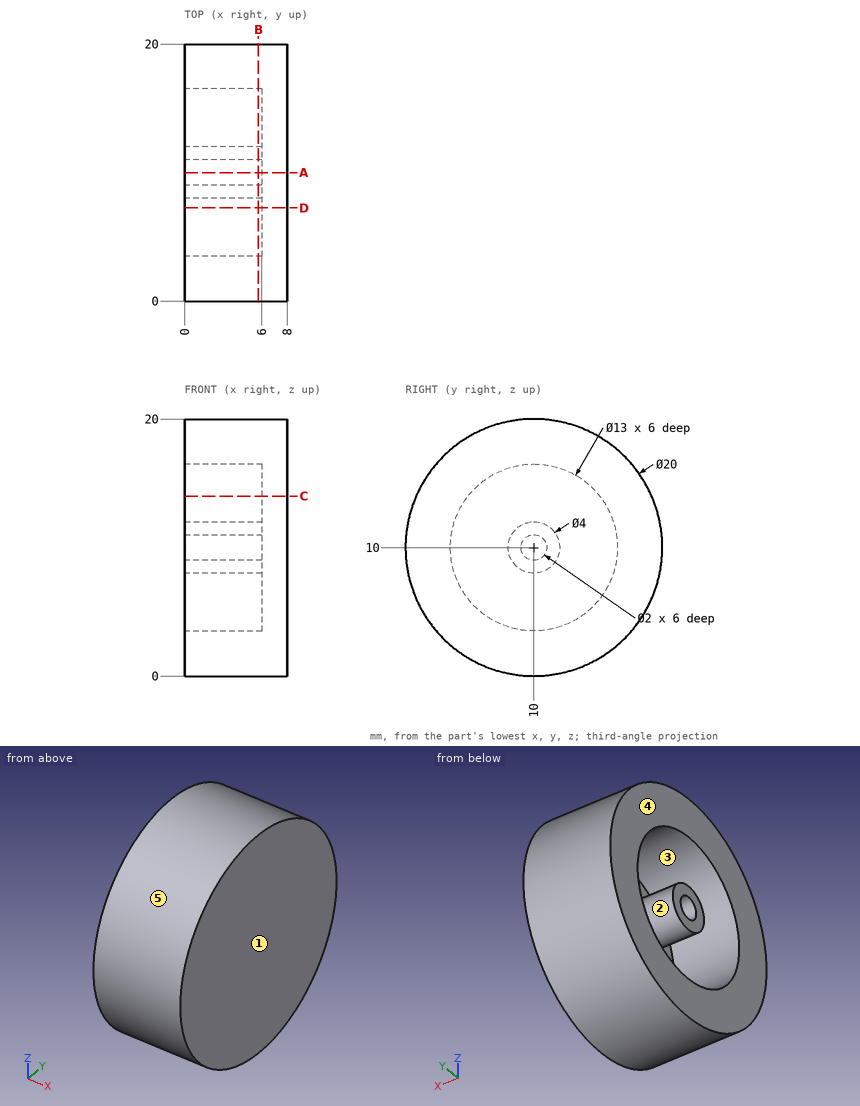
The figure shows three views and two pictorial views of one solid part (mm, origin at its lowest corner). Answer the questions. A direction names the side the tool comes from. Coordinates: 2 decimals unless noted, no trailing zeros. Order: outer loops, then holes, each group sorted by start corner. A loop starts at its lowest first (then second) coordinate and runs counter-clockwise, first axis right, second up. Notation, with made-up numbers: M 47,26 L 104,26 A7 cw 104,30 Z; hole C 69,-18.5 d4. An arc over 180 degrees is marked long. Use CSV: the item, a comma, the result in double quotes.
1) Section C-C on z = 14 is taken. Write down the section's boundary in (x, y), plus the area to 3 significant figures.
Worked out:
outline,"M 0,0.83 L 8,0.83 L 8,19.17 L 0,19.17 L 0,15.12 L 6,15.12 L 6,4.88 L 0,4.88 Z"
area,"85.2 mm^2"
2) Section B-B on x = 5.75 is taken. Write down the section's boundary in (y, z), plus the area to 3 significant figures.
Worked out:
outline,"C 10,10 d20; C 10,10 d4; hole C 10,10 d13; hole C 10,10 d2"
area,"191 mm^2"
3) Section A-A on y = 10 is taken. Write down the section's boundary in (x, z), plus the area to 3 significant figures.
Worked out:
outline,"M 0,0 L 8,0 L 8,20 L 0,20 L 0,16.5 L 6,16.5 L 6,12 L 0,12 L 0,11 L 6,11 L 6,9 L 0,9 L 0,8 L 6,8 L 6,3.5 L 0,3.5 Z"
area,"94.0 mm^2"
4) Consider line 1 (Y direction, x = 3.55, z = 10); line 2 (Y direction, x = 1.5, z = 8.75); line 3 (Z direction, x = 4.75, y = 8.25). Determine where each line is inside the solid, lowest interval first. Write a range as [from, to].
Worked out:
line 1,"y = [0, 3.5], [8, 9], [11, 12], [16.5, 20]"
line 2,"y = [0.08, 3.62], [8.44, 11.56], [16.38, 19.92]"
line 3,"z = [0.15, 3.74], [9.03, 10.97], [16.26, 19.85]"
5) For the marked faces 1 and 2, determine the directions among +Z, -Z, +X, -X, +Y, -Y from which every point of the face is accessible in a straight line to the end or side of a thin tool.
Worked out:
face 1,"+Z, -Z, +X, +Y, -Y"
face 2,"-X"
6) Determine the mould class of the marked faces 3, 4 and 5 for opening direction Z: released by +Z, released by -Z, zero draft, split by the parting line, or undercut.
Worked out:
face 3,"undercut"
face 4,"zero draft"
face 5,"split by the parting line"
7) Flat-ended cylindrical pins translate along their axes: pin 1 Ø1.5 at (x, y) = (2.5, 14) entering from -Z; pin 2 Ø2 at (x, y) = (2.5, 12) entering from +Z; pin 3 Ø2 at (x, y) = (3.5, 7) entering from +Z. Find the tip coordinate at first contact, or state that the pin passes through.
Worked out:
pin 1,"stops at z = 0.54"
pin 2,"stops at z = 19.95"
pin 3,"stops at z = 19.8"
8) Section D-D on y = 7.25 is taken. Write down the section's boundary in (x, z), plus the area to 3 significant figures.
Worked out:
outline,"M 0,0.39 L 8,0.39 L 8,19.61 L 0,19.61 L 0,15.89 L 6,15.89 L 6,4.11 L 0,4.11 Z"
area,"83.2 mm^2"
